from build123d import *

# Parameters (mm, degrees)
EXTRUDE_360_DEPTH = 1.4
SKETCH_4_W        = 0.2
SKETCH_4_H        = 10.309401077
CHAMFER_1921_SIZE = 0.32
FILLET_1966_R     = 0.1


with BuildPart() as part:
    # 草图1 → Extrude 360 (new body)
    with BuildSketch(Plane(origin=(0, 0, 0), x_dir=(0, 0, -1), z_dir=(1, 0, 0))):
        Polygon((2, 1.154700538), (2, -1.154700538), (0, -2.309401077), (-2, -1.154700538), (-2, 1.154700538), (0, 2.309401077), align=None)
    extrude(amount=EXTRUDE_360_DEPTH)

    # 草图2 → 凸台-旋转1 (revolve)
    with BuildSketch(Plane.XY, mode=Mode.PRIVATE) as revolve_1_sk:
        Polygon((0, 0), (36.4, 0), (36.4, 0.6536), (36.4, 1), (0, 1), align=None)
    revolve(revolve_1_sk.sketch.rotate(Axis((0, 0, 0), (1, 0, 0)), 90), axis=Axis((0, 0, 0), (1, 0, 0)))

    # 草图3 → 切除-旋转1 (revolve, cut)
    with BuildSketch(Plane.XY):
        Polygon((0, 2), (3.065384141, 7.309401077), (3.065384141, 12.309401077), (-10, 12.309401077), (-10, 2), align=None)
    revolve(axis=Axis((0, 0, 0), (1, 0, 0)), mode=Mode.SUBTRACT)

    # 草图5 → 切除-旋转2 (revolve, cut)
    with BuildSketch(Plane.XY):
        Polygon((1.4, 2), (-1.665384141, 7.309401077), (-1.665384141, 12.309401077), (8.334615859, 12.309401077), (8.334615859, 2), align=None)
    revolve(axis=Axis((0, 0, 0), (1, 0, 0)), mode=Mode.SUBTRACT)

    # 草图4 → 切除-旋转3 (revolve, cut)
    with BuildSketch(Plane.XY, mode=Mode.PRIVATE) as cut_revolve_3_sk:
        with Locations((1.3, 7.154700539)):
            Rectangle(SKETCH_4_W, SKETCH_4_H)
    revolve(cut_revolve_3_sk.sketch.rotate(Axis((0, 0, 0), (1, 0, 0)), 270), axis=Axis((0, 0, 0), (1, 0, 0)), mode=Mode.SUBTRACT)

    # Chamfer 1921
    chamfer_1921_edges = [part.edges().sort_by_distance(p)[0] for p in [
        (36.4, 0, -1),
    ]]
    chamfer(chamfer_1921_edges, length=CHAMFER_1921_SIZE)

    # Fillet 1966
    fillet_1966_edges = [part.edges().sort_by_distance(p)[0] for p in [
        (1.4, 0, -1),
    ]]
    fillet(fillet_1966_edges, radius=FILLET_1966_R)


solid = part.part
Design review of the part built by this model. Coordinates are the model's own, in mm. A direction names the side the tool comes from. Round coordinates to 2 decimals unless told otherwise and drop trailing zeros. Write each loop counter-clockwise with the first axis right and the second up, starting at its lowest first coordinate (ties: lowest second). Pieces come first, ordered by that corner, then holes. Notation, with made-up numbers: (39, 83.5) - (69, 83.5) arc R23 cw to (69, 121.5) - close; hole circle Ø8 at (44.25, 60). An arc over 180 degrees is marked (long way). Return JSON: item names as keys, results as strings. Group by question number.
Item 1: Machinability: for faces 1 (the face through (0.592, 1.724, 1.014)), 2 (the face through (1.4, -1, 1)), which of the approach directions +Z, -Z, +X, -X, +Y, -Y give a long, thin tool a straight path to every point of the face, cutting with its end or side? Answer none if there is none.
Item 2: For probe 1 along Y at (x, z) = (25.5, -0.1); probe 2 along X at (y, z) = (0.75, -1.15); probe 3 along Z at (x, y) = (12.5, -0.4), list the stretches that pass through material, from the lowest coordinate up. Write a range as [from, to].
Item 3: We need section A-A on x = 9.5. Write out the cut boundary in (y, z), and give its area (3 significant figures).
Item 4: Insertion check: P1, Ø2, axis at x = 4, z = 0, coming from the +Y side; P2, Ø1.5, axis at x = 8, z = 0, coming from the -Y side; P3, Ø0.8, axis at y = 1, z = 1.5, coming from the +X side. Each pin has a flat end and moves straight along its axis. Give the tip position at first contact, or say it passes through.
Model answer:
{
 "1": {"face 1": "+Z, +X, -X, +Y", "face 2": "+X"},
 "2": {"probe 1": "y = [-0.99, 0.99]", "probe 2": "x = [0, 1.4]", "probe 3": "z = [-0.92, 0.92]"},
 "3": {"outline": "circle Ø2 at (0, 0)", "area": "3.14 mm²"},
 "4": {"P1": "stops at y = 1", "P2": "stops at y = -1", "P3": "stops at x = 1.4"}
}
